The figure shows three views and two pictorial views of one solid part (mm, origin at its lowest corner). Answer the questions. Coordinates: 2 decimals unless noted, no trailing zeros. Order: outer loops, then holes, each group sorted by start corner. A loop starts at its lowest first (then second) coordinate and runs counter-clockwise, first axis right, second up. Notation, with made-up numbers: (-23.5, 87) - (-13.5, 87) arc R16 ccw to (-13.5, 109) - close; hole circle Ø7 at (5, 84.5). An arc over 180 degrees is marked (long way). Use one line per item in the form item = value.
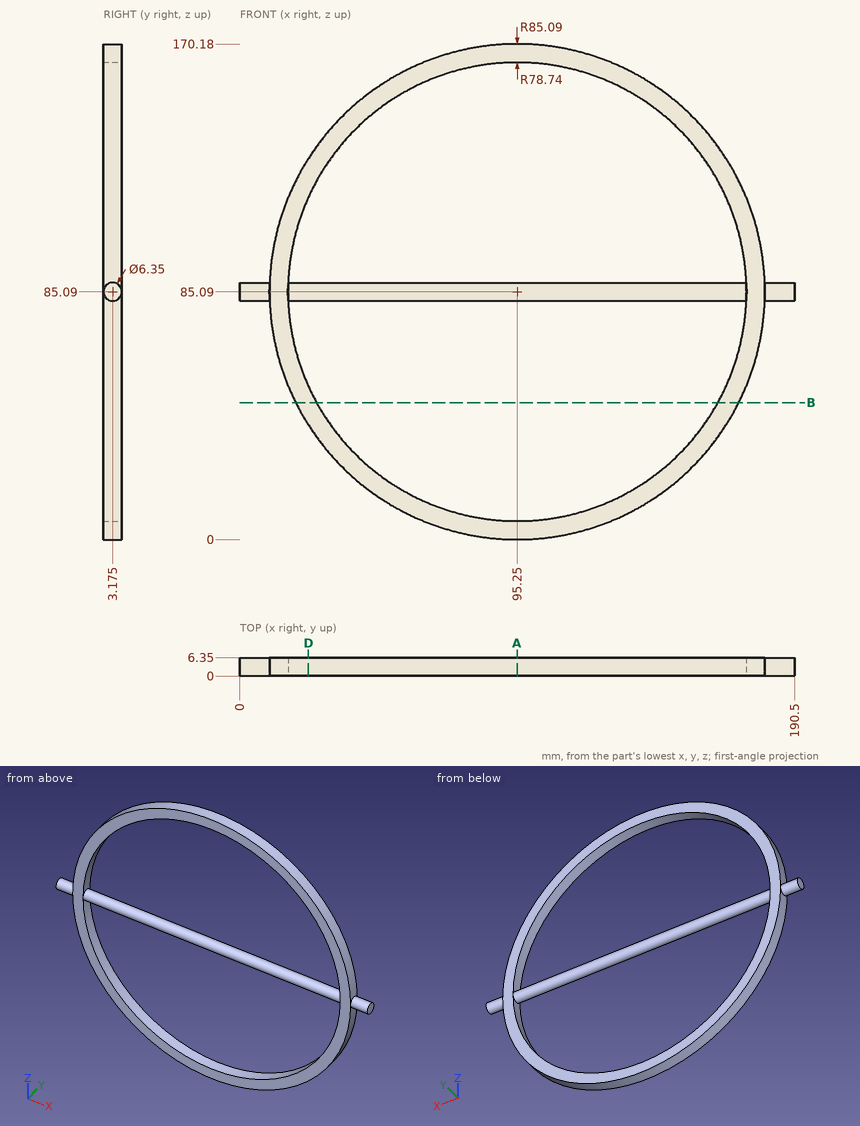
(1) Section A-A, the plane x = 95.25 is taken. Write down the section's boundary in (y, z) (3 decimals), then the cut area to 3 significant figures.
Answer list:
outline = (0, 0) - (6.35, 0) - (6.35, 6.35) - (0, 6.35) - close; circle Ø6.35 at (3.175, 85.09); (0, 163.83) - (6.35, 163.83) - (6.35, 170.18) - (0, 170.18) - close
area = 112 mm2
(2) Given pin 1 Ø2 at (x, y) = (138.5, 4.5) entering from -Z; pin 2 Ø1 at (x, y) = (27.5, 1) entering from -Z; pin 3 Ø2 at (x, y) = (69, 2.5) entering from -Z, each flat-ended and moving along its own axis, determine where each tip first touches the part or whether it passes through.
Answer list:
pin_1 = 11.23
pin_2 = 32.96
pin_3 = 3.83
(3) Straight lines are drawn through the part: L1, parallel to Z at x = 134, y = 3; L2, parallel to Z at x = 69.5, y = 4; L3, parallel to X at y = 0.5, z = 73. For each, find the intervals that lie inside material, in ascending order.
Answer list:
L1 = 9.34 to 16.54, 81.92 to 88.26, 153.64 to 160.84
L2 = 3.99 to 10.68, 82.02 to 88.16, 159.5 to 166.19
L3 = 11.02 to 17.44, 173.06 to 179.48
(4) Section B-B, the plane z = 47 is taken. Write down the section's boundary in (x, y), then the cut area to 3 significant figures.
Answer list:
outline = (19.16, 0) - (26.34, 0) - (26.34, 6.35) - (19.16, 6.35) - close; (164.16, 0) - (171.34, 0) - (171.34, 6.35) - (164.16, 6.35) - close
area = 91.1 mm2
(5) Section D-D, the plane x = 23.5 is taken. Write down the section's boundary in (y, z) (3 decimals).
Answer list:
outline = (0, 39.349) - (6.35, 39.349) - (6.35, 52.657) - (0, 52.657) - close; circle Ø6.35 at (3.175, 85.09); (0, 117.523) - (6.35, 117.523) - (6.35, 130.831) - (0, 130.831) - close
